```python
from build123d import *

# Parameters (mm, degrees)
SKETCH_R   = 3
SKETCH_R_2 = 4.15
PAD_DEPTH  = 4


with BuildPart() as part:
    # Sketch → Pad (new body, symmetric)
    with BuildSketch(Plane.XY):
        with BuildLine():
            Line((0, 8), (24, 8))
            ThreePointArc((26, 6), (25.414214, 7.414214), (24, 8))
            Line((26, 6), (26, -6))
            ThreePointArc((24, -8), (25.414214, -7.414214), (26, -6))
            Line((24, -8), (0, -8))
            ThreePointArc((0, 8), (-8, 0), (0, -8))
        make_face()
        with Locations((18.5, 0)):
            Circle(SKETCH_R, mode=Mode.SUBTRACT)
        Circle(SKETCH_R_2, mode=Mode.SUBTRACT)
    extrude(amount=PAD_DEPTH, both=True)


solid = part.part
```
Geometry check sheet. Reference: the model listing, model coordinates, mm. Round coordinates to 2 decimals unless told otherwise and drop trailing zeros. Loops run counter-clockwise (first coordinate to the right, second up) from the corner with the lowest first, then second, coordinate; pieces in that order, holes last. Notation, with made-up numbers: (-4.75, -27.5) - (3.25, -27.5) arc R20 ccw to (3.25, 11.5) - close; hole circle Ø6 at (75.25, -4.5). An arc over 180 degrees is marked (long way). Use a Markdown table: item, result.
Q1. Cross-section at A-A on x = 18.5. Record the cut outline in (y, z), plus the area to 3 significant figures.
Solutions:
| item | result |
|---|---|
| outline | (-8, -4) - (-3, -4) - (-3, 4) - (-8, 4) - close; (3, -4) - (8, -4) - (8, 4) - (3, 4) - close |
| area | 80.0 mm2 |
Q2. Cross-section at B-B on y = 0. Record the cut outline in (x, z), plus the area to 3 significant figures.
Solutions:
| item | result |
|---|---|
| outline | (-8, -4) - (-4.15, -4) - (-4.15, 4) - (-8, 4) - close; (4.15, -4) - (15.5, -4) - (15.5, 4) - (4.15, 4) - close; (21.5, -4) - (26, -4) - (26, 4) - (21.5, 4) - close |
| area | 158 mm2 |
Q3. Cross-section at D-D on x = -2.5. Record the cut outline in (y, z).
Solutions:
| item | result |
|---|---|
| outline | (-7.6, -4) - (-3.31, -4) - (-3.31, 4) - (-7.6, 4) - close; (3.31, -4) - (7.6, -4) - (7.6, 4) - (3.31, 4) - close |
Q4. Material ranges on line 1 (Y direction, x = 18.5, z = -1.5); line 2 (Y direction, x = 0, z = -1.25); line 3 (X direction, y = 2.5, z = 3.5), recorded low to high.
Solutions:
| item | result |
|---|---|
| line 1 | y = -8 to -3, 3 to 8 |
| line 2 | y = -8 to -4.15, 4.15 to 8 |
| line 3 | x = -7.6 to -3.31, 3.31 to 16.84, 20.16 to 26 |
Q5. Cross-section at C-C on z = -0.5. Record the cut outline in (x, y).
Solutions:
| item | result |
|---|---|
| outline | (0, -8) - (24, -8) arc R2 ccw to (26, -6) - (26, 6) arc R2 ccw to (24, 8) - (0, 8) arc R8 ccw to start; hole circle Ø8.3 at (0, 0); hole circle Ø6 at (18.5, 0) |
Q6. Go/stop test with flat-tipped pins: P1, Ø1, axis at y = -5.5, z = -0.5, coming from the -X side (3 decimals); P2, Ø4, axis at y = -3, z = -2.5, coming from the -X side. Record where each tip stops, or that it passes through.
Solutions:
| item | result |
|---|---|
| P1 | stops at x = -6.245 |
| P2 | stops at x = -7.94 |
Q7. Draft check along Y on faces 1 (the flat face through (12, 8, 0)), 2 (the cylindrical face through (-8, 0, 0)), 3 (the cylindrical face through (16.1, -1.8, -0.1)). Enter one of: released by +Y, released by -Y, zero draft, split by the parting line, or undercut.
Solutions:
| item | result |
|---|---|
| face 1 | released by +Y |
| face 2 | split by the parting line |
| face 3 | undercut |
